```python
from build123d import *

# Parameters (mm, degrees)
SKETCH1_R           = 79.4
SKETCH1_R_2         = 72.4
BOSS_EXTRUDE1_DEPTH = 0.6
SKETCH1_3_R         = 72.4
SKETCH1_3_R_2       = 70.4
BOSS_EXTRUDE2_DEPTH = 6
BOSS_EXTRUDE3_DEPTH = 3


with BuildPart() as part:
    # Sketch1 → Boss-Extrude1 (new body)
    with BuildSketch(Plane.XY):
        Circle(SKETCH1_R)
        Circle(SKETCH1_R_2, mode=Mode.SUBTRACT)
    extrude(amount=BOSS_EXTRUDE1_DEPTH)

    # Sketch1_3 → Boss-Extrude2 (add)
    with BuildSketch(Plane.XY):
        with BuildLine():
            Line((-6.182652597, 79.158921208), (-6.182652597, 81.164861898))
            ThreePointArc((-6.182652597, 81.164861898), (3.187118264, -81.337582194), (-0.187253418, 81.39978462))
            Line((-0.187253418, 81.39978462), (-0.182652597, 79.399789912))
            ThreePointArc((-0.182652597, 79.399789912), (3.184930452, -79.336096564), (-6.182652597, 79.158921208))
        make_face()
        Circle(SKETCH1_3_R)
        Circle(SKETCH1_3_R_2, mode=Mode.SUBTRACT)
    extrude(amount=BOSS_EXTRUDE2_DEPTH)

    # Sketch1_4 → Boss-Extrude3 (add)
    with BuildSketch(Plane.XY):
        with BuildLine():
            ThreePointArc((-0.187253418, 81.39978462), (-3.187118264, 81.337582194), (-6.182652597, 81.164861898))
            Line((-6.182652597, 81.164861898), (-6.182652597, 79.158921208))
            ThreePointArc((-6.182652597, 79.158921208), (-3.184930452, 79.336096564), (-0.182652597, 79.399789912))
            Line((-0.182652597, 79.399789912), (-0.187253418, 81.39978462))
        make_face()
        with BuildLine():
            Line((-6.182652597, 79.158921208), (-6.182652597, 81.164861898))
            ThreePointArc((-6.182652597, 81.164861898), (-55.329431945, -59.704388119), (81.4, 0))
            ThreePointArc((81.4, 0), (57.49224979, 57.624658039), (-0.187253418, 81.39978462))
            Line((-0.187253418, 81.39978462), (-0.182652597, 79.399789912))
            ThreePointArc((-0.182652597, 79.399789912), (56.0796638, 56.208818775), (79.4, 0))
            ThreePointArc((79.4, 0), (-53.91408621, -58.289204044), (-6.182652597, 79.158921208))
        make_face()
    extrude(amount=BOSS_EXTRUDE3_DEPTH)


solid = part.part
```
Could you check a few things on this model? Use its own coordinates, in mm. A direction names the side the tool comes from. Round coordinates to 2 decimals unless told otherwise and drop trailing zeros. Loops run counter-clockwise (first coordinate to the right, second up) from the corner with the lowest first, then second, coordinate; pieces in that order, holes last. Notation, with made-up numbers: (-16.75, -7.75) -> (30.25, -7.75) arc R14 cw to (30.25, -1.75) -> close; hole circle Ø8 at (33, 79). An arc over 180 degrees is marked (long way). One line per question, with ' | ' between items.
(1) For pin 1 Ø1 at (x, z) = (-10.5, 1.5) entering from -Y; pin 2 Ø2.5 at (x, y) = (-4, 80.5) entering from +Z; pin 3 Ø1.5 at (y, z) = (17.5, 5) entering from -X, each with a flat end and sliding along its axis, tell me the tip position at first contact or that it passes through.
Model answer:
pin 1: stops at y = -80.78 | pin 2: stops at z = 3 | pin 3: stops at x = -79.66
(2) If we section it at B-B on y = 0: List the corners of the cut face in (x, z) for me, and give its area (3 significant figures).
Model answer:
outline: (-81.4, 0) -> (-70.4, 0) -> (-70.4, 6) -> (-72.4, 6) -> (-72.4, 0.6) -> (-79.4, 0.6) -> (-79.4, 6) -> (-81.4, 6) -> close; (70.4, 0) -> (81.4, 0) -> (81.4, 6) -> (79.4, 6) -> (79.4, 0.6) -> (72.4, 0.6) -> (72.4, 6) -> (70.4, 6) -> close | area: 56.4 mm^2
(3) For faces 1 (the face through (69.057, 21.747, 3.262)), 2 (the face through (-37, 61, 0)), which set-ups out of +Z, -Z, +X, -X, +Y, -Y let a thin tool reach every point of the face, with its end or its side?
Model answer:
face 1: +Z | face 2: -Z, +X, -X, +Y, -Y
(4) Thinking about a two-plate mould opening in Y: for faces 3 (the face through (35, -64, 0.6)), 4 (the face through (16, -69, 6)), which applies, released by +Y, released by -Y, zero draft, split by the parting line, or undercut?
Model answer:
face 3: undercut | face 4: zero draft
(5) If I drill on probe 1 along Y at (x, z) = (1, 4.15); probe 2 along Y at (x, z) = (45.5, 4.2); probe 3 along X at (y, z) = (-12, 3.6), over which ranges is the centre line in solid material (lowest first)?
Model answer:
probe 1: y = -81.39 to -79.39, -72.39 to -70.39, 70.39 to 72.39, 79.39 to 81.39 | probe 2: y = -67.5 to -65.07, -56.32 to -53.72, 53.72 to 56.32, 65.07 to 67.5 | probe 3: x = -80.51 to -78.49, -71.4 to -69.37, 69.37 to 71.4, 78.49 to 80.51
(6) If we section it at A-A on z = 4.8: List the corners of the cut face in (x, y) for me, and give its area (3 significant figures).
Model answer:
outline: circle Ø144.8 at (0, 0); (-6.18, 79.16) -> (-6.18, 81.16) arc R81.4 ccw (long way) to (-0.19, 81.4) -> (-0.18, 79.4) arc R79.4 cw (long way) to start; hole circle Ø140.8 at (0, 0) | area: 1,900 mm^2
(7) If we section it at C-C on x = 17: List the corners of the cut face in (y, z) for me, and give its area (3 significant figures).
Model answer:
outline: (-79.61, 0) -> (-68.32, 0) -> (-68.32, 6) -> (-70.38, 6) -> (-70.38, 0.6) -> (-77.56, 0.6) -> (-77.56, 6) -> (-79.61, 6) -> close; (68.32, 0) -> (79.61, 0) -> (79.61, 6) -> (77.56, 6) -> (77.56, 0.6) -> (70.38, 0.6) -> (70.38, 6) -> (68.32, 6) -> close | area: 57.9 mm^2
